```python
from build123d import *

# Parameters (mm, degrees)
EXTRUDE_1_DEPTH     = 10
SKETCH_2_R          = 9.75
EXTRUDE_2_DEPTH     = 5
FILLET_2_R          = 1
SKETCH_3_R          = 5.6
CUT_EXTRUDE_1_DEPTH = 5


with BuildPart() as part:
    # 草图1 → 凸台-拉伸1 (new body)
    with BuildSketch(Plane.XY):
        with BuildLine():
            Line((-7.25, 2.4999999999999996), (7.249999999999998, 2.500000000000002))
            ThreePointArc((7.249999999999998, 2.500000000000002), (9.75, 4.33e-15), (7.250000000000002, -2.499999999999997))
            Line((7.250000000000002, -2.499999999999997), (-7.25, -2.4999999999999996))
            ThreePointArc((-7.25, -2.4999999999999996), (-9.75, 3.1e-16), (-7.25, 2.4999999999999996))
        make_face()
    extrude(amount=EXTRUDE_1_DEPTH)

    # 草图2 → 凸台-拉伸2 (add)
    with BuildSketch(Plane(origin=(-4.5e-16, 2.500000000000001, 0), x_dir=(1, 1.7e-16, 0), z_dir=(-1.7e-16, 1, 0))):
        Circle(SKETCH_2_R)
    extrude(amount=-EXTRUDE_2_DEPTH)

    # 圆角2
    fillet_2_edges = [part.edges().sort_by_distance(p)[0] for p in [
        (8.387e-14, -2.499999999999999, -9.75),
        (8.304e-14, 2.500000000000001, -9.75),
    ]]
    fillet(fillet_2_edges, radius=FILLET_2_R)

    # 草图3 → 切除-拉伸1 (cut)
    with BuildSketch(Plane(origin=(-4.5e-16, 2.500000000000001, 0), x_dir=(1, 1.7e-16, 0), z_dir=(-1.7e-16, 1, 0))):
        with Locations(Location((0, 0, 0), (0, 0, 180))):
            Circle(SKETCH_3_R)
    extrude(amount=-CUT_EXTRUDE_1_DEPTH, mode=Mode.SUBTRACT)


solid = part.part
```
Could you check a few things on this model? Use its own coordinates, in mm. Coordinates: 2 decimals unless noted, no trailing zeros. Write each loop counter-clockwise with the first axis right and the second up, starting at its lowest first coordinate (ties: lowest second). Pieces come first, ordered by that corner, then holes. Notation, with made-up numbers: M -30,41 L -11,41 A30 ccw -11,72 Z; hole C -29.75,51.5 d4. An arc over 180 degrees is marked long. Answer as CSV lines item,"result". Start each with the question number.
1) We'd pull the mould along X, two halves only. Please class faces 1 (the cylindrical face through (-9.75, -0.05, 6.04)), 2 (the cylindrical face through (9.75, 0.05, 6.04)), 3 (the cylindrical face through (5.595, 0.035, 0.246)), 4 (the cylindrical face through (0.258, 0.021, -9.747)): +X half, -X half, draft (parallel to the pull), parting line (faces both ways), or undercut.
2) For P1, Ø10, axis at x = -3.5, z = 4, coming from the -Y side, with a flat end and sliding along its axis, tell me the tip position at first contact or that it passes through.
3) I want a section at C-C, the plane y = 2.1. Please give me the cut outline in (x, z).
4) Please list where these lines run through material, in increasing order: line 1 (Z direction, x = 0, y = -1.35); line 2 (Z direction, x = -2.25, y = -1.05); line 3 (X direction, y = 2, z = -1.5). Write a range as from..to.
5) I want a section at B-B, the plane y = 0. Please give me the cut outline in (x, z), and give its area (3 significant figures).
6) I want a section at A-A, the plane x = 0. Please give me the cut outline in (y, z).
Data:
1,face 1,"-X half"
1,face 2,"+X half"
1,face 3,"undercut"
1,face 4,"parting line"
2,P1,"stops at y = -2.5"
3,outline,"M -8.61,4.14 A9.55 ccw long 8.61,4.14 L 8.61,10 L -8.61,10 Z; hole C 0,0 d11.2"
4,line 1,"z = -9.75..-5.6, 5.6..10"
4,line 2,"z = -9.49..-5.13, 5.13..10"
4,line 3,"x = -9.5..-5.4, 5.4..9.5"
5,outline,"M -9.75,0 A9.75 ccw 9.75,0 L 9.75,10 L -9.75,10 Z; hole C 0,0 d11.2"
5,area,"246 mm^2"
6,outline,"M -2.5,-8.75 A1 ccw -1.5,-9.75 L 1.5,-9.75 A1 ccw 2.5,-8.75 L 2.5,-5.6 L -2.5,-5.6 Z; M -2.5,5.6 L 2.5,5.6 L 2.5,10 L -2.5,10 Z"
